Source: CAD feature listing. Evaluate the final solid. Frame: model axes, mm. A direction names the side the tool comes from. Coordinates: 2 decimals unless noted, no trailing zeros. Write each loop counter-clockwise with the first axis right and the second up, starting at its lowest first coordinate (ties: lowest second). Pieces come first, ordered by that corner, then holes. Notation, with made-up numbers: M 32,11 L 87,11 A11 cw 87,32 Z; hole C -1,33.5 d5. An arc over 180 degrees is marked long. One line per item, written item: value. Start each with the question number.
Item 1: Pin query (flat end, axial travel): P1, Ø1.9, axis at y = -1.5, z = 37, coming from the -X side; P2, Ø1.9, axis at x = 28.5, y = -2.5, coming from the +Z side. Return the tip coordinate at first contact, or that it passes through.
Item 2: Set-up query: faces 1 (the flat face through (26.67, -3, 38)), 2 (the flat face through (30, -3, 0)), 3 (the flat face through (33.02, -3, 13)), 4 (the flat face through (-30, -3, 0)), 5 (the flat face through (-30, -3, 25.4)). Return all of +Z, -Z, +X, -X, +Y, -Y with unobstructed straight access to the full face (end or side cutting, diameter ignored); none if empty.
Item 3: Cut plane A-A, the plane y = -2.25. Output: boundary loops of the cut face in (x, z), then the cut area to 3 significant figures.
Item 4: Ray query, L1, parallel to Z at x = 30.5, y = -0.75; L2, parallel to X at y = -3.25, z = -10.5. Return the intervals inside material, ascending. Write a range as from..to.
Item 5: Mould query, pull axis Z, two halves, no side actions, for faces 6 (the flat face through (30, -3, -25.4)), 7 (the flat face through (30, -3, 25.4)), 8 (the flat face through (0, -3, -50.8)), 9 (the flat face through (33.02, -3, -38)). Classes: released by +Z, released by -Z, zero draft, split by the parting line, or undercut.
Item 6: Cut plane B-B, the plane z = 37. Output: boundary loops of the cut face in (x, y), then the cut area to 3 significant figures.
```python
from build123d import *

# Parameters (mm, degrees)
F0_W     = 6.35
F0_H     = 25.4
F1_DEPTH = 6.35


with BuildPart() as f1:
    # F0 (on Front) → F1 (new body)
    with BuildSketch(Plane.XZ):
        with Locations((-29.845, 12.7)):
            Rectangle(F0_W, F0_H)
        Polygon((-26.67, -50.8), (26.67, -50.8), (26.67, -25.4), (26.67, 0), (26.67, 25.4), (26.67, 50.8), (-26.67, 50.8), (-26.67, 25.4), (-26.67, 0), (-26.67, -25.4), align=None)
        with Locations((29.845, 12.7)):
            Rectangle(F0_W, F0_H)
        with Locations((29.845, -38.1)):
            Rectangle(F0_W, F0_H)
        with Locations((-29.845, -38.1)):
            Rectangle(F0_W, F0_H)
    extrude(amount=F1_DEPTH)


solid = f1.part
```
From the geometry:
1. P1: stops at x = -26.67
1. P2: stops at z = 25.4
2. face 1: +Z, +X, +Y, -Y
2. face 2: +X, +Y, -Y
2. face 3: +Z, -Z, +X, +Y, -Y
2. face 4: -X, +Y, -Y
2. face 5: +Z, -X, +Y, -Y
3. outline: M -33.02,-50.8 L 33.02,-50.8 L 33.02,-25.4 L 26.67,-25.4 L 26.67,0 L 33.02,0 L 33.02,25.4 L 26.67,25.4 L 26.67,50.8 L -26.67,50.8 L -26.67,25.4 L -33.02,25.4 L -33.02,0 L -26.67,0 L -26.67,-25.4 L -33.02,-25.4 Z
3. area: 6,060 mm²
4. L1: z = -50.8..-25.4, 0..25.4
4. L2: x = -26.67..26.67
5. face 6: undercut
5. face 7: released by +Z
5. face 8: released by -Z
5. face 9: zero draft
6. outline: M -26.67,-6.35 L 26.67,-6.35 L 26.67,0 L -26.67,0 Z
6. area: 339 mm²
